Geometry check sheet. Reference: the model listing, model coordinates, mm. A direction names the side the tool comes from. Round coordinates to 2 decimals unless told otherwise and drop trailing zeros. Loops run counter-clockwise (first coordinate to the right, second up) from the corner with the lowest first, then second, coordinate; pieces in that order, holes last.
```python
from build123d import *

# Parameters (mm, degrees)
EXTRUDE_428_DEPTH      = 5
EXTRUDE_428_DEPTH_BACK = 5
SKETCH_1_W             = 60
SKETCH_1_H             = 40
SKETCH_5_R             = 1.25
CUT_EXTRUDE_682_DEPTH  = 51.249378106
CUT_EXTRUDE_1222_DEPTH = 38.416573868
SKETCH_7_W             = 40
SKETCH_7_H             = 36
CUT_EXTRUDE_1460_DEPTH = 2.5
FILLET_1_R             = 1
FILLET_2_R             = 1
CHAMFER_1_SIZE         = 1


with BuildPart() as part:
    # Эскиз1 → Extrude 428 (new, two sides: drawn at the far end of the back side and taken through both)
    with BuildSketch(Plane(origin=(0, 0, 0), x_dir=(1, 0, 0), z_dir=(0, 1, 0)).offset(-EXTRUDE_428_DEPTH_BACK)):
        Rectangle(SKETCH_1_W, SKETCH_1_H)
    extrude(amount=EXTRUDE_428_DEPTH + EXTRUDE_428_DEPTH_BACK)

    # Эскиз5 → Cut-Extrude 682 (cut, through all)
    with BuildSketch(Plane.XY.offset(20)):
        with Locations((-25, 0)):
            Circle(SKETCH_5_R)
        with Locations((25, 0)):
            Circle(SKETCH_5_R)
    extrude(amount=-CUT_EXTRUDE_682_DEPTH, mode=Mode.SUBTRACT)

    # Эскиз6 → Cut-Extrude 1222 (cut, through all)
    with BuildSketch(Plane(origin=(0, 5, 0), x_dir=(1, 0, 0), z_dir=(0, 1, 0))):
        Polygon((-18.505152884, 18), (18.505152884, 18), (0, 1.345362405), align=None)
        Polygon((20, 16.654637595), (20, -16.654637595), (1.494847116, 0), align=None)
        Polygon((-18.505152884, -18), (18.505152884, -18), (0, -1.345362405), align=None)
        Polygon((-20, 16.654637595), (-20, -16.654637595), (-1.494847116, 0), align=None)
    extrude(amount=-CUT_EXTRUDE_1222_DEPTH, mode=Mode.SUBTRACT)

    # Эскиз7 → Cut-Extrude 1460 (cut)
    with BuildSketch(Plane(origin=(0, 5, 0), x_dir=(1, 0, 0), z_dir=(0, 1, 0))):
        Rectangle(SKETCH_7_W, SKETCH_7_H)
    cut_extrude_1460 = extrude(amount=-CUT_EXTRUDE_1460_DEPTH, mode=Mode.SUBTRACT)

    # Зеркальное отражение1: Cut-Extrude 1460 across plane
    add(cut_extrude_1460.mirror(Plane.ZX), mode=Mode.SUBTRACT)

    # Скругление1
    fillet_1_edges = [part.edges().sort_by_distance(p)[0] for p in [
        (18.505152884, 0, 18),
        (-18.505152884, 0, 18),
        (-20, 0, 16.654637595),
        (-20, 0, -16.654637595),
        (-18.505152884, 0, -18),
        (18.505152884, 0, -18),
        (20, 0, -16.654637595),
        (20, 0, 16.654637595),
        (-20, -3.75, -18),
        (-20, -3.75, 18),
        (20, -3.75, 18),
        (20, -3.75, -18),
        (20, 3.75, -18),
        (-20, 3.75, -18),
        (-20, 3.75, 18),
        (20, 3.75, 18),
    ]]
    fillet(fillet_1_edges, radius=FILLET_1_R)

    # Скругление2
    fillet_2_edges = [part.edges().sort_by_distance(p)[0] for p in [
        (0, 0, 1.345362405),
        (-1.494847116, 0, 0),
        (0, 0, -1.345362405),
        (1.494847116, 0, 0),
    ]]
    fillet(fillet_2_edges, radius=FILLET_2_R)

    # Фаска1
    chamfer_1_edges = [part.edges().sort_by_distance(p)[0] for p in [
        (30, -5, 0),
        (-30, 5, 0),
        (30, 5, 0),
        (-30, -5, 0),
    ]]
    chamfer(chamfer_1_edges, length=CHAMFER_1_SIZE)


solid = part.part
```
1) Sectioned sample at A-A, the plane x = 0. Record the cut outline in (y, z), then the cut area to 3 significant figures.
Report:
outline: (-5, -20) - (5, -20) - (5, -18) - (-5, -18) - close; (-5, 18) - (5, 18) - (5, 20) - (-5, 20) - close; (-2.5, -1.69) - (2.5, -1.69) - (2.5, 1.69) - (-2.5, 1.69) - close
area: 56.9 mm2
2) Gauge pin test, flat end, axial feed: pin 1 (5 mm diameter, centred on x = 16.5, z = -14.5, fed in from -Y). Record the tip position at first contact, or that the pin passes through.
Report:
pin 1: stops at y = -2.5
3) Access from +Z, -Z, +X, -X, +Y, -Y to the whole of each face (thin tool, end or side, straight path). Record for faces 3 (the face through (-23.845, -0.479, 0.28)), 4 (the face through (-8.507, 0.035, 9.002)).
Report:
face 3: +Z, -Z
face 4: +Y, -Y
4) Sectioned sample at B-B, the plane z = -11.5. Record the cut outline in (x, y).
Report:
outline: (-30, -4) - (-29, -5) - (-20, -5) - (-20, 5) - (-29, 5) - (-30, 4) - close; (-14.27, -2.5) - (-11.28, -2.5) - (-11.28, 2.5) - (-14.27, 2.5) - close; (11.28, -2.5) - (14.27, -2.5) - (14.27, 2.5) - (11.28, 2.5) - close; (20, -5) - (29, -5) - (30, -4) - (30, 4) - (29, 5) - (20, 5) - close; hole circle Ø2.5 at (-25, 0); hole circle Ø2.5 at (25, 0)
5) Sectioned sample at C-C, the plane x = 25. Record the cut outline in (y, z).
Report:
outline: (-5, -20) - (-1.25, -20) - (-1.25, 20) - (-5, 20) - close; (1.25, -20) - (5, -20) - (5, 20) - (1.25, 20) - close
6) Sectioned sample at D-D, the plane y = 0. State how many separate pieces and enclosed holes the cut face has, then the cut area to 3 significant figures.
Report:
separate pieces: 3
enclosed holes: 4
area: 978 mm2
7) Scan lines: line 1 along Z through (x, y) = (15, -1); line 2 along Z through (x, y) = (4, 3); line 3 along Z through (x, y) = (11, -1.5). Record each from-to range of solid material in increasing order.
Report:
line 1: z = -20 to -18, -14.85 to -12.15, 12.15 to 14.85, 18 to 20
line 2: z = -20 to -18, 18 to 20
line 3: z = -20 to -18, -11.25 to -8.55, 8.55 to 11.25, 18 to 20
8) Mould release check, pull along X, two halves, no side actions. Record for faces 1 (the face through (0, 0, -20)), 2 (the face through (0.01, -0.04, 1.69)): +X half, -X half, draft (parallel to the pull), parting line (faces both ways), or undercut.
Report:
face 1: draft
face 2: undercut
